CAD build for the part. Positions are in the model's coordinates, mm. A direction names the side the tool comes from. Round coordinates to 2 decimals unless told otherwise and drop trailing zeros. Loops run counter-clockwise (first coordinate to the right, second up) from the corner with the lowest first, then second, coordinate; pieces in that order, holes last.
Autodesk Inventor part; units mm, degrees
ref_plane "Work Plane1" through (4.4, 8, -54.5) normal (1, 0, 0) x (0, 0, -1)
ref_plane "Work Plane2" through (-39.2, 8, -19.1) normal (0, 0, -1) x (-1, 0, 0)
ref_plane "YZ Plane" through (0, 0, 0) normal (1, 0, 0) x (0, 1, 0)
sketch "Sketch1" plane through (0, 0, 0) normal (0, 1, 0) x (-1, 0, 0)
  line L0 (38, 0) -> (0, 0)
  line L1 (0, 0) -> (0, -45)
  line L2 (0, -45) -> (-8, -45)
  line L3 (-8, -45) -> (-63, -49.5)
  line L4 (-63, -49.5) -> (-63, -79)
  line L5 (-63, -79) -> (-46, -96)
  line L6 (-46, -96) -> (3, -96)
  line L7 (3, -96) -> (55, -44)
  line L8 (55, -44) -> (55, -17)
  line L9 (55, -17) -> (38, 0)
  line L10 (19, -15) -> (39.2, -15)
  line L11 (39.2, -15) -> (39.2, -23.2)
  line L12 (39.2, -23.2) -> (19, -23.2)
  line L13 (19, -23.2) -> (19, -15)
  line L14 (-0.3, -68) -> (-8.5, -68)
  line L15 (-8.5, -68) -> (-8.5, -83.5)
  line L16 (-8.5, -83.5) -> (-0.3, -83.5)
  line L17 (-0.3, -83.5) -> (-0.3, -68)
  dimension "d0" = 45
  dimension "d1" = 55
  dimension "d2" = 63
  dimension "d3" = 96
  dimension "d4" = 8
  dimension "d6" = 45
  dimension "d7" = 45
  dimension "d8" = 45
  dimension "d9" = 46.5
  dimension "d10" = 17
  dimension "d11" = 44
  dimension "d12" = 17
  dimension "d13" = 8.2
  dimension "d14" = 20.2
  dimension "d15" = 8.2
  dimension "d16" = 15.5
  dimension "d17" = 12.5
  dimension "d18" = 19
  dimension "d19" = 15
  dimension "d20" = 54.5
extrude "Extrusion1" add sketch "Sketch1" along normal blind 8
fillet "Fillet1" radius 15 6 edges at (-38, 4, 0) (-55, 4, -17) (-55, 4, -44) (-3, 4, -96) (46, 4, -96) (63, 4, -79)
fillet "Fillet2" radius 5 1 edges at (63, 4, -49.5)
sketch "Sketch2" plane through (0, 8, 0) normal (0, 1, 0) x (1, 0, 0)
  arc A0 (58.4077, 49.1243) -> (63, 54.1076) centre (58, 54.1076) ccw construction
  line L0 (63, 54.1076) -> (63, 72.7868) construction
  arc A1 (63, 72.7868) -> (58.6066, 83.3934) centre (48, 72.7868) ccw construction
  line L1 (58.6066, 83.3934) -> (50.3934, 91.6066) construction
  arc A2 (50.3934, 91.6066) -> (39.7868, 96) centre (39.7868, 81) ccw construction
  line L2 (39.7868, 96) -> (3.2132, 96) construction
  arc A3 (3.2132, 96) -> (-7.3934, 91.6066) centre (3.2132, 81) ccw construction
  line L3 (-7.3934, 91.6066) -> (-50.6066, 48.3934) construction
  arc A4 (-50.6066, 48.3934) -> (-55, 37.7868) centre (-40, 37.7868) ccw construction
  line L4 (-55, 37.7868) -> (-55, 23.2132) construction
  arc A5 (-55, 23.2132) -> (-50.6066, 12.6066) centre (-40, 23.2132) ccw construction
  line L5 (-50.6066, 12.6066) -> (-42.3934, 4.3934) construction
  arc A6 (-42.3934, 4.3934) -> (-31.7868, 0) centre (-31.7868, 15) ccw construction
  line L6 (-31.7868, 0) -> (0, 0) construction
  line L7 (0, 0) -> (0, 45) construction
  line L8 (0, 45) -> (8, 45) construction
  line L9 (8, 45) -> (58.4077, 49.1243) construction
  line L10 (0.3, 68) -> (0.3, 83.5) construction
  line L11 (0.3, 83.5) -> (8.5, 83.5) construction
  line L12 (8.5, 83.5) -> (8.5, 68) construction
  line L13 (8.5, 68) -> (0.3, 68) construction
  line L14 (-39.2, 15) -> (-39.2, 23.2) construction
  line L15 (-39.2, 23.2) -> (-19, 23.2) construction
  line L16 (-19, 23.2) -> (-19, 15) construction
  line L17 (-19, 15) -> (-39.2, 15) construction
  line L18 (-39.2, 23.2) -> (-39.2, 15) construction
  line L19 (-39.2, 19.1) -> (-44.7, 19.1) construction
  line L20 (4.4, 54.5) -> (4.4, 68) construction
  line L21 (0.3, 68) -> (8.5, 68) construction
  line L22 (43.5, 78.5) -> (43.5, 57) construction
  line L23 (-39.2, 15) -> (-39.2, 23.2) construction
  line L24 (8.5, 68) -> (0.3, 68) construction
  point P0 (28, 70)
  dimension "d25" = 5.5
  dimension "d26" = 13.5
  dimension "d27" = 26
  dimension "d28" = 35
  dimension "d29" = 19.5
  dimension "d30" = 17.5
  dimension "d31" = 39
hole "Hole1" at (28, 8, -70) at (4.4, 8, -54.5) at (-44.7, 8, -19.1) direction (0, -1, 0) diameter 3.5 end through all
hole "Hole2" at (43.5, 8, -78.5) direction (0, -1, 0) diameter 8 end through all
hole "Hole3" at (43.5, 8, -57) direction (0, -1, 0) diameter 10 end through all
ref_plane "Work Plane1" through (4.4, 8, -54.5) normal (1, 0, 0) x (0, 0, -1)
ref_plane "Work Plane2" through (-39.2, 8, -19.1) normal (0, 0, -1) x (-1, 0, 0)
properties part number "A8-0004"
Item 1: Cut at B-B, the plane x = 28. Give the cut face in (y, z), plus the area to 3 significant figures.
Answers follow:
outline: (0, -96) - (8, -96) - (8, -71.75) - (0, -71.75) - close; (0, -68.25) - (8, -68.25) - (8, -46.64) - (0, -46.64) - close
area: 367 mm2
Item 2: Cut at C-C, the plane z = -19.1. Give the cut face in (x, y), plus the area to 3 significant figures.
Answers follow:
outline: (-54.43, 0) - (-46.45, 0) - (-46.45, 8) - (-54.43, 8) - close; (-42.95, 0) - (-39.2, 0) - (-39.2, 8) - (-42.95, 8) - close; (-19, 0) - (0, 0) - (0, 8) - (-19, 8) - close
area: 246 mm2
Item 3: Flat gauge pins, fed straight in: P1, Ø1, axis at x = -39, z = -14, coming from the -Y side; P2, Ø2.5, axis at y = 3, z = -25, coming from the +X side; P3, Ø2.5, axis at y = 4, z = -73.5, coming from the -X side; P4, Ø2.5, axis at y = 3, z = -78, coming from the +X side. Where does each tip first touch, or does it go through?
Answers follow:
P1: stops at y = 0
P2: stops at x = 0
P3: stops at x = -26.75
P4: stops at x = 62.47
Item 4: Cut at D-D, the plane x = 43.5. Give the cut face in (y, z).
Answers follow:
outline: (0, -95.53) - (8, -95.53) - (8, -82.5) - (0, -82.5) - close; (0, -74.5) - (8, -74.5) - (8, -62) - (0, -62) - close; (0, -52) - (8, -52) - (8, -47.9) - (0, -47.9) - close
Item 5: Cut at A-A, the plane y = 2.25. State how many separate pieces and enclosed holes the cut face has, plus the area to 3 significant figures.
Answers follow:
separate pieces: 1
enclosed holes: 7
area: 6,240 mm2
Item 6: 3-axis set-ups, long thin cutter, end or side, ignore diameter. For faces 1 (the flat face through (63, 4, -63)), 2 (the flat face through (0, 4, -22)), 3 (the flat face through (4, 4, -83.5)): which of +Z, -Z, +X, -X, +Y, -Y reach the whole face in a straight line?
Answers follow:
face 1: +Z, -Z, +X, +Y, -Y
face 2: +Z, +X, +Y, -Y
face 3: +Y, -Y
Item 7: Probe line 1 (Z direction, x = 4.4, y = 1.5); line 2 (X direction, y = 2.75, z = -70); line 3 (Z direction, x = 43.5, y = 5). List the from-to ranges inside material, lowest first.
Answers follow:
line 1: z = -96 to -83.5, -68 to -56.25, -52.75 to -45
line 2: x = -29 to 0.3, 8.5 to 26.25, 29.75 to 63
line 3: z = -95.53 to -82.5, -74.5 to -62, -52 to -47.9
Item 8: Two-plate mould, pull along Z, no slides. Class faces 4 (the flat face through (4, 4, -45)), 5 (the flat face through (5, 8, -47)), 6 (the flat face through (-29, 4, -23.2)): released by +Z, released by -Z, zero draft, split by the parting line, or undercut.
Answers follow:
face 4: released by +Z
face 5: zero draft
face 6: undercut
